Can you work these out from the model? Positions are in its coordinate system, mm. Face numbers are marked on the shaded views. A direction names the side the tool comes from. Give positions to 0.01 mm unless a question says otherwise; leave off trailing zeros. Write each loop counter-clockwise with the first axis right and the second up, starting at its lowest first coordinate (ties: lowest second). Pieces come first, ordered by that corner, then holes.
1. Suppose I cut it at B-B (y = 7.75). Please give me the cut outline in (x, z), and give its area (3 significant figures).
2. Suppose I cut it at A-A (x = 0). Please give me the cut outline in (y, z).
3. If I drill on probe 1 along X at (y, z) = (6, -4.75); probe 2 along Z at (x, y) = (-1.75, 3.25); probe 3 along X at (y, z) = (2, 1.5), over which ranges is the centre line in solid material (lowest first)?
4. I'm going to push flat-ended pins straight in: pin 1 (4.5 mm diameter, centred on x = -0.5, z = -0.5, fed in from -Y); pin 2 (1.4 mm diameter, centred on y = 4, z = -4, fed in from +X); pin 3 (1 mm diameter, centred on y = 2.5, z = 1, fed in from +X); pin 4 (1.5 mm diameter, centred on y = 1.5, z = -1.5, fed in from +X). Where does each tip first touch, or does it pass through?
5. On a 3-axis mill with a long thin cutter (end or side, diameter ignored), from which of +Z, -Z, +X, -X, +Y, -Y can I reach the whole of each face in a straight line? I mean the marked faces 4, 5 and 6. Say none if no direction works.
6. Suppose I cut it at C-C (z = 1). Please give me the cut outline in (x, y), and give its area (3 significant figures).
7. Thinking about a two-plate mould opening in Z: for the marked faces 1, 2 and 3, which applies, pulls with the +Z half, pulls with the -Z half, needs draft (parallel to the pull), parting line crosses it, or undercut?
8. Suppose I cut it at D-D (x = -1). Please give me the cut outline in (y, z).
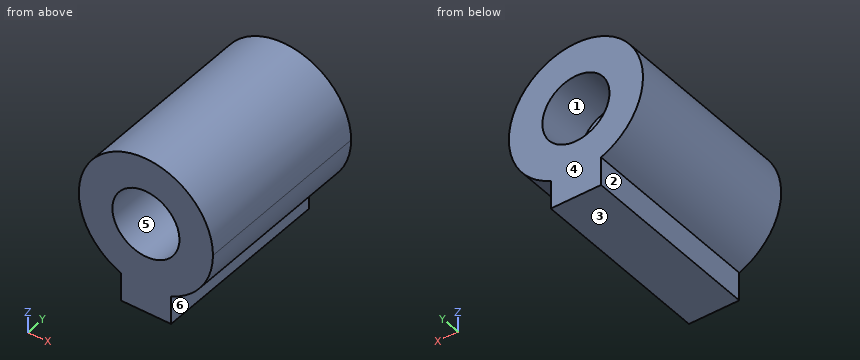
```python
from build123d import *

# Parameters (mm, degrees)
EXTRUDE_3_DEPTH     = 10
EXTRUDE_4_DEPTH     = 1
SKETCH_6_R          = 2
CUT_EXTRUDE_1_DEPTH = 3
EXTRUDE_5_DEPTH     = 1
CUT_EXTRUDE_START   = -7
SKETCH_9_R          = 2
CUT_EXTRUDE_3_DEPTH = 7
SKETCH_10_R         = 0.5
CUT_EXTRUDE_5_DEPTH = 10.703607577


with BuildPart() as part:
    # 草图4 → 凸台-拉伸3 (new body)
    with BuildSketch(Plane(origin=(0, 0, 0), x_dir=(1, 0, 0), z_dir=(0, 1, 0))):
        with BuildLine():
            Line((-1.5, 3.708099244), (-1.5, 0))
            Line((-1.5, 0), (1.5, 0))
            Line((1.5, 0), (1.5, 3.708099244))
            ThreePointArc((1.5, 3.708099244), (0, 4), (-1.5, 3.708099244))
        make_face()
        with BuildLine():
            Line((1.5, 0), (-1.5, 0))
            Line((-1.5, 0), (-1.5, 3.708099244))
            ThreePointArc((-1.5, 3.708099244), (-2.236067977, -3.31662479), (4, 0))
            ThreePointArc((4, 0), (3.31662479, 2.236067977), (1.5, 3.708099244))
            Line((1.5, 3.708099244), (1.5, 0))
        make_face()
        with BuildLine():
            Line((-1.5, 3.708099244), (-1.5, 0))
            Line((-1.5, 0), (1.5, 0))
            Line((1.5, 0), (1.5, 3.708099244))
            ThreePointArc((1.5, 3.708099244), (0, 4), (-1.5, 3.708099244))
        make_face()
        with BuildLine():
            Line((1.5, 0), (-1.5, 0))
            Line((-1.5, 0), (-1.5, 3.708099244))
            ThreePointArc((-1.5, 3.708099244), (-2.236067977, -3.31662479), (4, 0))
            ThreePointArc((4, 0), (3.31662479, 2.236067977), (1.5, 3.708099244))
            Line((1.5, 3.708099244), (1.5, 0))
        make_face()
        with BuildLine():
            Line((-1.5, 5.4), (-1.5, 3.708099244))
            ThreePointArc((-1.5, 3.708099244), (0, 4), (1.5, 3.708099244))
            Line((1.5, 3.708099244), (1.5, 5.4))
            Line((1.5, 5.4), (-1.5, 5.4))
        make_face()
    extrude(amount=EXTRUDE_3_DEPTH)

    # 草图5 → 凸台-拉伸4 (add)
    with BuildSketch(Plane(origin=(0, 10, 0), x_dir=(1, 0, 0), z_dir=(0, 1, 0))):
        with BuildLine():
            ThreePointArc((4, 0), (3.31662479, 2.236067977), (1.5, 3.708099244))
            ThreePointArc((1.5, 3.708099244), (0, 4), (-1.5, 3.708099244))
            ThreePointArc((-1.5, 3.708099244), (-2.236067977, -3.31662479), (4, 0))
        make_face()
    extrude(amount=EXTRUDE_4_DEPTH)

    # 草图6 → 切除-拉伸1 (cut)
    with BuildSketch(Plane(origin=(0, 11, 0), x_dir=(1, 0, 0), z_dir=(0, 1, 0))):
        with Locations(Location((0, 0, 0), (0, 0, 270))):
            Circle(SKETCH_6_R)
    extrude(amount=-CUT_EXTRUDE_1_DEPTH, mode=Mode.SUBTRACT)

    # 草图7 → 凸台-拉伸5 (add)
    with BuildSketch(Plane(origin=(0, 10, 0), x_dir=(1, 0, 0), z_dir=(0, 1, 0))):
        with BuildLine():
            ThreePointArc((-1.5, 3.708099244), (0, 4), (1.5, 3.708099244))
            Line((1.5, 3.708099244), (1.5, 5.4))
            Line((1.5, 5.4), (-1.5, 5.4))
            Line((-1.5, 5.4), (-1.5, 3.708099244))
        make_face()
    extrude(amount=EXTRUDE_5_DEPTH)

    # 草图9 → 切除-拉伸3 (cut)
    with BuildSketch(Plane.XZ.offset(CUT_EXTRUDE_START)):
        with Locations(Location((0, 0, 0), (0, 0, 90))):
            Circle(SKETCH_9_R)
    extrude(amount=CUT_EXTRUDE_3_DEPTH, mode=Mode.SUBTRACT)

    # 草图10 → 切除-拉伸5 (cut, through all)
    with BuildSketch(Plane.XZ.offset(-7)):
        with Locations(Location((0, 0, 0), (0, 0, 270))):
            Circle(SKETCH_10_R)
    extrude(amount=-CUT_EXTRUDE_5_DEPTH, mode=Mode.SUBTRACT)


solid = part.part
```
Checks:
1. outline: (-1.5, -5.4) - (1.5, -5.4) - (1.5, -3.71) arc R4 ccw (long way) to (-1.5, -3.71) - close; hole circle Ø1 at (0, 0)
1. area: 54.0 mm2
2. outline: (0, -5.4) - (11, -5.4) - (11, -2) - (8, -2) - (8, -0.5) - (7, -0.5) - (7, -2) - (0, -2) - close; (0, 2) - (7, 2) - (7, 0.5) - (8, 0.5) - (8, 2) - (11, 2) - (11, 4) - (0, 4) - close
3. probe 1: x = -1.5 to 1.5
3. probe 2: z = -3.6 to -0.97, 0.97 to 3.6
3. probe 3: x = -3.71 to -1.32, 1.32 to 3.71
4. pin 1: stops at y = 0
4. pin 2: stops at x = 2.26
4. pin 3: stops at x = 3.97
4. pin 4: stops at x = 3.93
5. face 4: +Z, -Z, +X, -X, +Y
5. face 5: -Y
5. face 6: -Z, +X, +Y, -Y
6. outline: (-3.87, 0) - (-1.73, 0) - (-1.73, 7) - (1.73, 7) - (1.73, 0) - (3.87, 0) - (3.87, 11) - (1.73, 11) - (1.73, 8) - (-1.73, 8) - (-1.73, 11) - (-3.87, 11) - close
6. area: 50.6 mm2
7. face 1: undercut
7. face 2: needs draft
7. face 3: pulls with the -Z half
8. outline: (0, -5.4) - (11, -5.4) - (11, -1.73) - (8, -1.73) - (8, 1.73) - (11, 1.73) - (11, 3.87) - (0, 3.87) - (0, 1.73) - (7, 1.73) - (7, -1.73) - (0, -1.73) - close
